from build123d import *

# Parameters (mm, degrees)
F0_W     = 290
F0_H     = 40
F0_W_2   = 254
F0_H_2   = 7
F1_DEPTH = 15
F2_W     = 254
F2_H     = 10.7
F3_DEPTH = 10
F4_R     = 3.3
F5_DEPTH = 15


with BuildPart() as f1:
    # F0 (on Top) → F1 (new body)
    with BuildSketch(Plane.XY):
        Rectangle(F0_W, F0_H)
        Rectangle(F0_W_2, F0_H_2, mode=Mode.SUBTRACT)
    extrude(amount=F1_DEPTH)

    # F2 (on face) → F3 (cut)
    with BuildSketch(Plane.XY.offset(15)):
        Rectangle(F2_W, F2_H)
    extrude(amount=-F3_DEPTH, mode=Mode.SUBTRACT)

    # F4 (on face) → F5 (cut, through all)
    with BuildSketch(Plane(origin=(0, 0, 0), x_dir=(1, 0, 0), z_dir=(0, 0, -1))):
        with Locations((-136, 0)):
            Circle(F4_R)
        with Locations((136, 0)):
            Circle(F4_R)
    extrude(amount=-F5_DEPTH, mode=Mode.SUBTRACT)


solid = f1.part
Work out the finished part from the listing and answer in its coordinate system (mm). A direction names the side the tool comes from. Coordinates: 2 decimals unless noted, no trailing zeros. Loops run counter-clockwise (first coordinate to the right, second up) from the corner with the lowest first, then second, coordinate; pieces in that order, holes last. Notation, with made-up numbers: M 64.5,44 L 89.5,44 A37 ccw 89.5,81 Z; hole C -15,13 d3. An arc over 180 degrees is marked long. Answer in a Markdown table with one row per item. Add a question column.
1. The mould has two halves that part along X. Classify faces 4 (the flat face through (127, 0, 7)), 5 (the flat face through (-145, 0, 7)), 6 (the flat face through (-2, -20, 7)): pulls with the +X half, pulls with the -X half, needs draft (parallel to the pull), parting line crosses it, or undercut.
2. Consider L1, parallel to X at y = 0, z = 3.75; L2, parallel to Y at x = -110.5, z = 3.25; L3, parallel to Y at x = 136, z = 9.5. Determine where each line is inside the solid, lowest interval first.
3. Find section B-B, the plane y = 0. Write down the section's boundary in (x, z).
4. Find section D-D, the plane x = 136. Write down the section's boundary in (y, z).
5. Find section A-A, the plane x = 100.5. Write down the section's boundary in (y, z), then the cut area to 3 significant figures.
6. A tool of negligible diameter and unlimited length cuts with its end or side. For faces 1 (the flat face through (-2, 9, 15)), 2 (the flat face through (-2, -3.5, 2)), 3 (the flat face through (-2, -5.35, 10)), from which of +Z, -Z, +X, -X, +Y, -Y can it reach the whole face along a straight path? Write none if from no direction.
7. Find section C-C, the plane z = 2.75. Write down the section's boundary in (x, y), then the cut area to 3 significant figures.
8. Flat-ended cylindrical pins translate along their axes: P1, Ø6, axis at x = -136, y = 0, coming from the -Z side; P2, Ø0.6, axis at x = -42, y = 4.5, coming from the +Z side. Find the tip coordinate at first contact, or state that the pin passes through.
Reported:
| question | item | result |
|---|---|---|
| 1 | face 4 | undercut |
| 1 | face 5 | pulls with the -X half |
| 1 | face 6 | needs draft |
| 2 | L1 | x = -145 to -139.3, -132.7 to -127, 127 to 132.7, 139.3 to 145 |
| 2 | L2 | y = -20 to -3.5, 3.5 to 20 |
| 2 | L3 | y = -20 to -3.3, 3.3 to 20 |
| 3 | outline | M -145,0 L -139.3,0 L -139.3,15 L -145,15 Z; M -132.7,0 L -127,0 L -127,15 L -132.7,15 Z; M 127,0 L 132.7,0 L 132.7,15 L 127,15 Z; M 139.3,0 L 145,0 L 145,15 L 139.3,15 Z |
| 4 | outline | M -20,0 L -3.3,0 L -3.3,15 L -20,15 Z; M 3.3,0 L 20,0 L 20,15 L 3.3,15 Z |
| 5 | outline | M -20,0 L -3.5,0 L -3.5,5 L -5.35,5 L -5.35,15 L -20,15 Z; M 3.5,0 L 20,0 L 20,15 L 5.35,15 L 5.35,5 L 3.5,5 Z |
| 5 | area | 458 mm^2 |
| 6 | face 1 | +Z, +X, -X, +Y, -Y |
| 6 | face 2 | +Z, -Z |
| 6 | face 3 | +Z |
| 7 | outline | M -145,-20 L 145,-20 L 145,20 L -145,20 Z; hole C -136,0 d6.6; hole M -127,-3.5 L 127,-3.5 L 127,3.5 L -127,3.5 Z; hole C 136,0 d6.6 |
| 7 | area | 9,750 mm^2 |
| 8 | P1 | passes through |
| 8 | P2 | stops at z = 5 |
